Model file for the job. Use its own axes, mm. A direction names the side the tool comes from. Round coordinates to 2 decimals unless told otherwise and drop trailing zeros. Order: outer loops, then holes, each group sorted by start corner. A loop starts at its lowest first (then second) coordinate and runs counter-clockwise, first axis right, second up. Notation, with made-up numbers: (80, -13) - (85, -13) arc R21 ccw to (85, 18) - close; hole circle Ø11 at (15, 19.5). An arc over 180 degrees is marked (long way). Put each result on its own line as item: value. Start each with the question number.
Item 1: Which spindle directions (+Z, -Z, +X, -X, +Y, -Y) get a long thin tool onto all of the face, cutting with end or side? Do faces 1 (the face through (5, 36, -12.7)), 2 (the face through (6.35, 71, -5)), 3 (the face through (27, 8.128, 0)). Say none if no direction does.
Item 2: Probe probe 1 along Z at (x, y) = (5, 107.95); probe 2 along X at (y, z) = (22.5, -5.5); probe 3 along Y at (x, z) = (39.5, -7.25). List the from-to ranges inside material, lowest first.
Item 3: Saw through at B-B on z = 0. List the corners of the cut face in (x, y), plus the area to 3 significant figures.
Item 4: Pin check, flat tips, straight feed: pin 1 Ø1.5 at (x, z) = (33, 6.5) entering from +Y; pin 2 Ø8 at (y, z) = (69.5, 2) entering from +X. Stop position of each tip, or through.
Item 5: Saw through at A-A on y = 69.85. List the corners of the cut face in (x, z).
Item 6: Mould opens along Y. For faces 4 (the face through (5, 36, 12.7)), 5 (the face through (3.131, 104.837, -0.98)), 6 (the face through (7.8, 15.48, 0.18)) say: pulls with the +Y half, pulls with the -Y half, needs draft (parallel to the pull), parting line crosses it, or undercut.
Item 7: Saw through at D-D on y = 86.5. List the corners of the cut face in (x, z), plus the area to 3 significant figures.
Item 8: Saw through at C-C on x = 5. List the corners of the cut face in (y, z), plus the area to 3 significant figures.
```python
from build123d import *

# Parameters (mm, degrees)
BOSS_EXTRUDE1_DEPTH = 12.7
SKETCH2_R           = 4.953
CUT_EXTRUDE1_DEPTH  = 138.371503595
CUT_EXTRUDE2_START  = 8.128
SKETCH3_R           = 11.1125
CUT_EXTRUDE2_DEPTH  = 130.243503595
SKETCH4_R           = 3.2639
CUT_EXTRUDE3_DEPTH  = 138.371503595


with BuildPart() as part:
    # Sketch1 → Boss-Extrude1 (new, symmetric)
    with BuildSketch(Plane.XY):
        with BuildLine():
            Line((0, 0), (0, 127))
            ThreePointArc((0, 127), (4.490128061, 125.140128061), (6.35, 120.65))
            Line((6.35, 120.65), (6.35, 19.51601695))
            ThreePointArc((6.35, 19.51601695), (7.835617786, 15.434315629), (11.597334072, 13.262487719))
            Line((11.597334072, 13.262487719), (44.546470768, 7.452665928))
            ThreePointArc((44.546470768, 7.452665928), (49.029509666, 4.864382214), (50.8, 0))
            Line((50.8, 0), (0, 0))
        make_face()
    extrude(amount=BOSS_EXTRUDE1_DEPTH, both=True)

    # Sketch2 → Cut-Extrude1 (cut, through all)
    with BuildSketch(Plane(origin=(0, 0, 0), x_dir=(1, 0, 0), z_dir=(0, 1, 0))):
        with Locations((33.3248, 0)):
            Circle(SKETCH2_R)
    extrude(amount=CUT_EXTRUDE1_DEPTH, mode=Mode.SUBTRACT)

    # Sketch3 → Cut-Extrude2 (cut, through all)
    with BuildSketch(Plane(origin=(0, 0, 0), x_dir=(1, 0, 0), z_dir=(0, 1, 0)).offset(CUT_EXTRUDE2_START)):
        with Locations((33.3248, 0)):
            Circle(SKETCH3_R)
    extrude(amount=CUT_EXTRUDE2_DEPTH, mode=Mode.SUBTRACT)

    # Sketch4 → Cut-Extrude3 (cut, through all)
    with BuildSketch(Plane(origin=(0, 0, 0), x_dir=(0, 0, -1), z_dir=(1, 0, 0))):
        with Locations(Location((0, 69.85, 0), (0, 0, 270))):
            Circle(SKETCH4_R)
        with Locations(Location((0, 107.95, 0), (0, 0, 270))):
            Circle(SKETCH4_R)
    extrude(amount=CUT_EXTRUDE3_DEPTH, mode=Mode.SUBTRACT)


solid = part.part
```
Results found:
1. face 1: -Z, +X, -X, +Y, -Y
1. face 2: +Z, -Z, +X, +Y
1. face 3: +Y
2. probe 1: z = -12.7 to -3.26, 3.26 to 12.7
2. probe 2: x = 0 to 6.35
2. probe 3: y = 0 to 8.13
3. outline: (0, 0) - (28.37, 0) - (28.37, 8.13) - (22.21, 8.13) - (22.21, 11.39) - (11.6, 13.26) arc R6.35 cw to (6.35, 19.52) - (6.35, 66.59) - (0, 66.59) - close; (0, 73.11) - (6.35, 73.11) - (6.35, 104.69) - (0, 104.69) - close; (0, 111.21) - (6.35, 111.21) - (6.35, 120.65) arc R6.35 ccw to (0, 127) - close; (38.28, 0) - (50.8, 0) arc R7.57 ccw to (44.55, 7.45) - (40.72, 8.13) - (38.28, 8.13) - close
3. area: 1,060 mm²
4. pin 1: stops at y = 8.13
4. pin 2: stops at x = 6.35
5. outline: (0, -12.7) - (6.35, -12.7) - (6.35, -3.26) - (0, -3.26) - close; (0, 3.26) - (6.35, 3.26) - (6.35, 12.7) - (0, 12.7) - close
6. face 4: needs draft
6. face 5: undercut
6. face 6: pulls with the +Y half
7. outline: (0, -12.7) - (6.35, -12.7) - (6.35, 12.7) - (0, 12.7) - close
7. area: 161 mm²
8. outline: (0, -12.7) - (124.56, -12.7) - (124.56, 12.7) - (0, 12.7) - close; hole circle Ø6.53 at (69.85, 0); hole circle Ø6.53 at (107.95, 0)
8. area: 3,100 mm²
